Build history of the part. All positions in model axes, mm. A direction names the side the tool comes from. Round coordinates to 2 decimals unless told otherwise and drop trailing zeros. Write each loop counter-clockwise with the first axis right and the second up, starting at its lowest first coordinate (ties: lowest second). Pieces come first, ordered by that corner, then holes.
1) Which spindle directions (+Z, -Z, +X, -X, +Y, -Y) get a long thin tool onto all of the face, cutting with end or side? Do faces 1 (the flat face through (-7.2, 5, 6)), 2 (the flat face through (0, 5, 12)), 3 (the cylindrical face through (0.98, 15.06, 9.1)), 4 (the flat face through (-5, 4.064, 6)). Say none if no direction does.
2) Flat gauge pins, fed straight in: pin 1 (2 mm diameter, centred on x = -1, y = 4.5, fed in from -Z); pin 2 (0.8 mm diameter, centred on y = 4.5, z = 7.5, fed in from +X); pin 3 (1.3 mm diameter, centred on y = 5, z = 4, fed in from -X). Where does each tip first touch, or does it go through?
3) Saw through at B-B (z = 11). State how many separate pieces and enclosed holes the cut face has, plus the area to 3 significant figures.
4) Pull direction X, two halves, no side cores. Call faces 5 (the flat face through (0, 5, 0)), 6 (the flat face through (0, 4.064, 6)), 7 (the flat face through (7.2, 5, 6)): +X half, -X half, draft (parallel to the pull), parting line (faces both ways), or undercut.
5) Saw through at A-A (y = 0). Write the cut outline in (x, z).
6) Saw through at C-C (y = 4.75). Write the cut outline in (x, z).
7) Wall check: probe 1 along X at (y, z) = (0, 9); probe 2 along Y at (x, z) = (-2.25, 11.5); probe 3 along Z at (x, y) = (-1.25, 4.25). Give the ranges that are in metal, low to high.
from build123d import *

# Parameters (mm, degrees)
SKETCH1_R           = 5.25
SKETCH1_R_2         = 4.5
BOSS_EXTRUDE1_DEPTH = 12
BOSS_EXTRUDE2_DEPTH = 2.54
SKETCH3_R           = 3.175
BOSS_EXTRUDE3_DEPTH = 2.54
BOSS_EXTRUDE3_DRAFT = -60
SKETCH4_R           = 3.25
BOSS_EXTRUDE4_DEPTH = 12


with BuildPart() as part:
    # Sketch1 → Boss-Extrude1 (new body)
    with BuildSketch(Plane.XY):
        Circle(SKETCH1_R)
        Circle(SKETCH1_R_2, mode=Mode.SUBTRACT)
    extrude(amount=BOSS_EXTRUDE1_DEPTH)

    # Sketch2 → Boss-Extrude2 (add)
    with BuildSketch(Plane(origin=(0, 4.064, 0), x_dir=(1, 0, 0), z_dir=(0, 1, 0))):
        Polygon((0, 0), (7.2, 0), (7.2, -12), (-7.2, -12), (-7.2, 0), align=None)
    extrude(amount=BOSS_EXTRUDE2_DEPTH)


with BuildPart() as boss_extrude3_tool:
    # Sketch3 → Boss-Extrude3 (with draft: the straight prism first)
    with BuildSketch(Plane(origin=(0, 6.604, 0), x_dir=(1, 0, 0), z_dir=(0, 1, 0))):
        with Locations((0, -6)):
            Circle(SKETCH3_R)
    extrude(amount=BOSS_EXTRUDE3_DEPTH)
    # Boss-Extrude3: the draft: its side faces are tilted about the plane it starts from
    boss_extrude3_sides = [boss_extrude3_tool.faces().sort_by_distance(p)[0] for p in [
        (-3.175, 7.874, 6),
    ]]
    draft(boss_extrude3_sides, Plane(origin=(0, 6.604, 0), x_dir=(1, 0, 0), z_dir=(0, 1, 0)), BOSS_EXTRUDE3_DRAFT)


with BuildPart() as part_1:
    add(part.part)

    # Boss-Extrude3: add boss_extrude3_tool
    add(boss_extrude3_tool.part)

    # Sketch4 → Boss-Extrude4 (add)
    with BuildSketch(Plane(origin=(0, 9.144, 0), x_dir=(1, 0, 0), z_dir=(0, 1, 0))):
        with Locations(Location((0, -6, 0), (0, 0, 270))):
            Circle(SKETCH4_R)
    extrude(amount=BOSS_EXTRUDE4_DEPTH)

    # Boss-Extrude5 cone 1 section (through the dimple's axis) → Boss-Extrude5 (revolve)
    with BuildSketch(Plane(origin=(0, 21.144, 6), x_dir=(0, 0, -1), z_dir=(1, 0, 0))):
        Polygon((0, 0), (3.25, 0), (0, 1.876388375), align=None)
    revolve(axis=Axis((0, 21.144, 6), (0, 1, 0)))


solid = part_1.part
Evaluation:
1. face 1: +Z, -Z, -X, -Y
1. face 2: +Z, +X, -X, -Y
1. face 3: +Y
1. face 4: +Z, -Z, -X
2. pin 1: stops at z = 0
2. pin 2: stops at x = 7.2
2. pin 3: stops at x = -7.2
3. separate pieces: 2
3. enclosed holes: 1
3. area: 66.1 mm2
4. face 5: draft
4. face 6: undercut
4. face 7: +X half
5. outline: (-5.25, 0) - (-4.5, 0) - (-4.5, 12) - (-5.25, 12) - close; (4.5, 0) - (5.25, 0) - (5.25, 12) - (4.5, 12) - close
6. outline: (-7.2, 0) - (7.2, 0) - (7.2, 12) - (-7.2, 12) - close
7. probe 1: x = -5.25 to -4.5, 4.5 to 5.25
7. probe 2: y = -4.74 to -3.9, 3.9 to 6.6, 8.2 to 9.14
7. probe 3: z = 0 to 12
